```python
from build123d import *

# Parameters (mm, degrees)
EXTRUDE_6_DEPTH          = 50
CUT_EXTRUDE_1_DEPTH      = 134.718463472
CUT_EXTRUDE_1_DEPTH_BACK = 134.718463472
SKETCH_5_R               = 21.601831088
CUT_EXTRUDE_2_DEPTH      = 99.714931123
SHELL_3_T                = -2


with BuildPart() as part:
    # 草图3 → 凸台-拉伸6 (new body)
    with BuildSketch(Plane(origin=(0, 0, 0), x_dir=(1, 0, 0), z_dir=(0, 1, 0))):
        with BuildLine():
            Line((-35.258285714, 30.485027968), (74.741714286, 30.485027968))
            ThreePointArc((74.741714286, 30.485027968), (78.277248192, 29.020561874), (79.741714286, 25.485027968))
            Line((79.741714286, 25.485027968), (79.741714286, -26.314972032))
            ThreePointArc((79.741714286, -26.314972032), (78.277248192, -29.850505938), (74.741714286, -31.314972032))
            Line((74.741714286, -31.314972032), (-35.258285714, -31.314972032))
            ThreePointArc((-35.258285714, -31.314972032), (-38.79381962, -29.850505938), (-40.258285714, -26.314972032))
            Line((-40.258285714, -26.314972032), (-40.258285714, 25.485027968))
            ThreePointArc((-40.258285714, 25.485027968), (-38.79381962, 29.020561874), (-35.258285714, 30.485027968))
        make_face()
    extrude(amount=EXTRUDE_6_DEPTH)

    # 草图4 → 切除-拉伸1 (cut, two sides: drawn at the far end of the back side and taken through both)
    with BuildSketch(Plane(origin=(79.741714286, 0, 0), x_dir=(0, 0, -1), z_dir=(1, 0, 0)).offset(-CUT_EXTRUDE_1_DEPTH_BACK)):
        Polygon((30.485027968, 50), (-31.314972032, 43), (-31.314972032, 50), align=None)
    extrude(amount=CUT_EXTRUDE_1_DEPTH + CUT_EXTRUDE_1_DEPTH_BACK, mode=Mode.SUBTRACT)

    # 草图5 → 切除-拉伸2 (cut, through all)
    with BuildSketch(Plane(origin=(0, 45.957380333, 5.205528517), x_dir=(1, 0, 0), z_dir=(0, 0.9936461847514532, 0.11254892060291542))):
        with Locations(Location((44.741714286, 3.723601101, 0), (0, 0, 270))):
            Circle(SKETCH_5_R)
        with Locations(Location((-5.258285714, 3.723601101, 0), (0, 0, 270))):
            Circle(SKETCH_5_R)
    extrude(amount=-CUT_EXTRUDE_2_DEPTH, mode=Mode.SUBTRACT)

    # 抽壳3
    shell_3_openings = [part.faces().sort_by_distance(p)[0] for p in [
        (-5.258285714, 24.353508562, -22.728886231),
        (44.741714286, 24.353508562, -22.728886231),
        (19.741714286, 0, 3.178829845),
    ]]
    offset(amount=SHELL_3_T, openings=shell_3_openings, kind=Kind.INTERSECTION)


solid = part.part
```
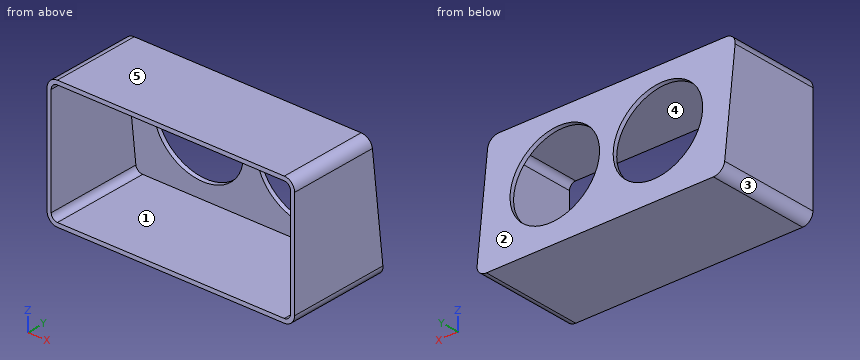
Part model, mm, in its own coordinate system. Face numbers are marked on the shaded views. A direction names the side the tool comes from. Coordinates: 2 decimals unless noted, no trailing zeros. Order: outer loops, then holes, each group sorted by start corner. A loop starts at its lowest first (then second) coordinate and runs counter-clockwise, first axis right, second up. Notation, with made-up numbers: (81.5, 62.25) - (92.5, 62.25) arc R12 ccw to (92.5, 66.25) - close; hole circle Ø3 at (58.25, 29). An arc over 180 degrees is marked (long way). Return JSON: item names as keys, results as strings. Group by question number.
Item 1: Drill centre lines: probe 1 along Z at (x, y) = (37.5, 2.5); probe 2 along X at (y, z) = (41.5, -2); probe 3 along Z at (x, y) = (49.5, 44.5). Where is each one in solid material? Low to high. Write a range as from..to.
Item 2: Pull direction X, two halves, no side cores. Call the marked faces 1, 2 and 3: pulls with the +X half, pulls with the -X half, needs draft (parallel to the pull), parting line crosses it, or undercut.
Item 3: Cut at B-B (x = 3). List the corners of the cut face in (y, z).
Item 4: Cut at D-D (x = 63). List the corners of the cut face in (y, z), plus the area to 3 significant figures.
Item 5: Which spindle directions (+Z, -Z, +X, -X, +Y, -Y) get a long thin tool onto all of the face, cutting with end or side? Do the marked faces 4 and 5. Say none if no direction does.
Item 6: Cut at C-C (z = -1). State how many separate pieces and enclosed holes the cut face has, plus the area to 3 significant figures.
Item 7: Cut at A-A (y = 29). List the corners of the cut face in (x, z).
Check values:
{
 "1": {"probe 1": "z = -30.49..-28.49, 29.31..31.31", "probe 2": "x = -40.26..-38.26, 77.74..79.74", "probe 3": "z = -30.49..-28.49"},
 "2": {"face 1": "undercut", "face 2": "needs draft", "face 3": "pulls with the -X half"},
 "3": {"outline": "(0, -30.49) - (50, -30.49) - (48.62, -18.33) - (46.64, -18.55) - (47.76, -28.49) - (0, -28.49) - close; (0, 29.31) - (41.21, 29.31) - (42.14, 21.11) - (44.13, 21.34) - (43, 31.31) - (0, 31.31) - close"},
 "4": {"outline": "(0, -30.49) - (50, -30.49) - (47.68, -9.97) - (45.69, -10.19) - (47.76, -28.49) - (0, -28.49) - close; (0, 29.31) - (41.21, 29.31) - (43.09, 12.75) - (45.08, 12.98) - (43, 31.31) - (0, 31.31) - close", "area": "256 mm2"},
 "5": {"face 4": "-Y", "face 5": "+Z, +X, -X, +Y, -Y"},
 "6": {"separate pieces": "3", "enclosed holes": "0", "area": "247 mm2"},
 "7": {"outline": "(-40.26, -25.49) arc R5 ccw to (-35.26, -30.49) - (74.74, -30.49) arc R5 ccw to (79.74, -25.49) - (79.74, 26.31) arc R5 ccw to (74.74, 31.31) - (-35.26, 31.31) arc R5 ccw to (-40.26, 26.31) - close; hole (-38.26, -25.49) arc R3 ccw to (-35.26, -28.49) - (74.74, -28.49) arc R3 ccw to (77.74, -25.49) - (77.74, 26.31) arc R3 ccw to (74.74, 29.31) - (-35.26, 29.31) arc R3 ccw to (-38.26, 26.31) - close"}
}
